Work out the finished part from the listing and answer in its coordinate system (mm). Round coordinates to 2 decimals unless told otherwise and drop trailing zeros. Order: outer loops, then holes, each group sorted by start corner. A loop starts at its lowest first (then second) coordinate and runs counter-clockwise, first axis right, second up. Notation, with made-up numbers: (-23, 27.5) - (13, 27.5) arc R22 cw to (13, 66.5) - close; hole circle Ø9 at (80.25, 71). An arc over 180 degrees is marked (long way). Use one line per item in the form item = value. Start each with the question number.
Q1. Given P1, Ø2.5, axis at x = 7, z = 0, coming from the -Y side; P2, Ø3, axis at y = 2.5, z = 4, coming from the -X side, each flat-ended and moving along its own axis, determine where each tip first touches the part or whether it passes through.
Q2. The part is cut by section C-C on x = -7. Determine the outline of the cut face in (y, z) (3 decimals), plus the area to 3 significant figures.
Q3. The part is cut by section B-B on y = 0.5. Determine the outline of the cut face in (x, z) (3 decimals).
Q4. The part is cut by section D-D on z = -3. Determine the outline of the cut face in (x, y).
Q5. For a pull along X with two mould halves and no side action, classify faces 1 (the cylindrical face through (0.2, 2.46, -8.51)), 2 (the cylindrical face through (2.38, 2.46, 10.74)), 3 (the flat face through (3, 5, 3)) as +X half, -X half, draft (parallel to the pull), parting line (faces both ways), or undercut.
Q6. Find the intervals of material crossed by line 1 (Z direction, x = 0, y = 3.2) (3 decimals); line 2 (X direction, y = 3.8, z = 7.5); line 3 (Z direction, x = 7, y = 1.9) (3 decimals), in increasing order. Write a range as [from, to].
Q7. The part is cut by section A-A on z = 0. Determine the outline of the cut face in (x, y) (3 decimals), plus the area to 3 significant figures.
Autodesk Inventor part; units mm, degrees
ref_plane "YZ Plane" through (0, 0, 0) normal (1, 0, 0) x (0, 1, 0)
ref_plane "XZ Plane" through (0, 0, 0) normal (0, 1, 0) x (-1, 0, 0)
ref_plane "XY Plane" through (0, 0, 0) normal (0, 0, 1) x (1, 0, 0)
sketch "草图1" plane through (0, 0, 0) normal (0, 1, 0) x (-1, 0, 0)
  circle A0 centre (0, 0) radius 11
  circle A1 centre (0, 0) radius 7
  circle A2 centre (0, 0) radius 3.5
  circle A3 centre (7, 0) radius 1.525
  circle A4 centre (0, 7) radius 1.525
  line L0 (0, 0) -> (2.2993, 0)
  line L1 (0, 0) -> (0, -1.9489)
  circle A5 centre (0, -7) radius 1.525
  circle A6 centre (-7, 0) radius 1.525
  dimension "d0" = 22
  dimension "d1" = 14
  dimension "d2" = 7
  dimension "d3" = 3.05
  dimension "d4" = 3.05
extrude "拉伸1" add sketch "草图1" along normal blind 5 contours A0 | A3 A1 A5 A6 A4
properties part number "leg5"
Found:
q1.P1 = through
q1.P2 = -10.71
q2.outline = (0, -8.485) - (5, -8.485) - (5, -1.525) - (0, -1.525) - close; (0, 1.525) - (5, 1.525) - (5, 8.485) - (0, 8.485) - close
q2.area = 69.6 mm²
q3.outline = circle Ø22 at (0, 0); hole circle Ø3.05 at (-7, 0); hole circle Ø7 at (0, 0); hole circle Ø3.05 at (0, -7); hole circle Ø3.05 at (0, 7); hole circle Ø3.05 at (7, 0)
q4.outline = (-10.58, 0) - (-1.8, 0) - (-1.8, 5) - (-10.58, 5) - close; (1.8, 0) - (10.58, 0) - (10.58, 5) - (1.8, 5) - close
q5.face_1 = undercut
q5.face_2 = parting line
q5.face_3 = draft
q6.line_1 = [-11, -8.525], [-5.475, -3.5], [3.5, 5.475], [8.525, 11]
q6.line_2 = [-8.05, -1.44], [1.44, 8.05]
q6.line_3 = [-8.485, -1.525], [1.525, 8.485]
q7.outline = (-11, 0) - (-8.525, 0) - (-8.525, 5) - (-11, 5) - close; (-5.475, 0) - (-3.5, 0) - (-3.5, 5) - (-5.475, 5) - close; (3.5, 0) - (5.475, 0) - (5.475, 5) - (3.5, 5) - close; (8.525, 0) - (11, 0) - (11, 5) - (8.525, 5) - close
q7.area = 44.5 mm²
